Geometry check sheet. Reference: the model listing, model coordinates, mm. A direction names the side the tool comes from. Give positions to 0.01 mm unless a question says otherwise; leave off trailing zeros. Loops run counter-clockwise (first coordinate to the right, second up) from the corner with the lowest first, then second, coordinate; pieces in that order, holes last. Notation, with made-up numbers: (-18.5, 83.5) -> (37.5, 83.5) arc R12 cw to (37.5, 105.5) -> close; hole circle Ø1 at (8.25, 66). An arc over 180 degrees is marked (long way). Answer as a JSON object with one key per item and string values.
from build123d import *

# Parameters (mm, degrees)
BOSS_EXTRUDE1_DEPTH = 10
SKETCH4_R           = 1.45
CUT_EXTRUDE2_DEPTH  = 93.209340633
FILLET3_R           = 5
CHAMFER1_SIZE       = 3
FILLET1_R           = 5
FILLET2_R           = 5
CHAMFER2_SIZE       = 1.6
CUT_EXTRUDE1_DEPTH  = 165.519185811
CHAMFER3_SIZE       = 1.6


# Some blends are built 0.0001 mm under size
with BuildPart() as part:
    # Sketch2 → Boss-Extrude1 (new body)
    with BuildSketch(Plane.XY):
        Polygon((-44.75, 78), (-37.75, 78), (-37.75, -74), (37.75, -74), (37.75, 78), (44.75, 78), (44.75, -80), (-44.75, -80), align=None)
    extrude(amount=BOSS_EXTRUDE1_DEPTH)

    # Sketch4 → Cut-Extrude2 (cut, through all)
    with BuildSketch(Plane.XY.offset(10)):
        with Locations((-41.25, 68)):
            Circle(SKETCH4_R)
        with Locations(Location((41.25, 68, 0), (0, 0, 180))):
            Circle(SKETCH4_R)
    extrude(amount=-CUT_EXTRUDE2_DEPTH, mode=Mode.SUBTRACT)

    # Fillet3
    fillet3_edges = [part.edges().sort_by_distance(p)[0] for p in [
        (-37.75, -74, 5),
        (37.75, -74, 5),
    ]]
    fillet(fillet3_edges, radius=FILLET3_R)

    # Chamfer1
    # the kernel refuses this chamfer: 3 mm, written as the material it takes off along each edge
    with BuildSketch(Plane(origin=(37.75, -69, 10), x_dir=(0.9996219169112968, 0, 0.02749587661058619), z_dir=(0, 1, 0))) as chamfer1_piece_1:
        Polygon((CHAMFER1_SIZE * 0.999621916911, CHAMFER1_SIZE * 0.0274958766106), (-CHAMFER1_SIZE * 0.0274958766106, CHAMFER1_SIZE * 0.999621916911), (0, 0), align=None)
    extrude(amount=154.715048964, mode=Mode.SUBTRACT)
    with BuildSketch(Plane(origin=(-32.75, -74, 10), x_dir=(0, -0.9996219169112968, 0.02749587661058619), z_dir=(1, 0, 0))) as chamfer1_piece_2:
        Polygon((CHAMFER1_SIZE * 0.999621916911, CHAMFER1_SIZE * 0.0274958766106), (-CHAMFER1_SIZE * 0.0274958766106, CHAMFER1_SIZE * 0.999621916911), (0, 0), align=None)
    extrude(amount=65.5, mode=Mode.SUBTRACT)
    with BuildSketch(Plane(origin=(-37.75, 85.715048964, 10), x_dir=(0.027495876610586775, 0, -0.9996219169112968), z_dir=(0, -1, 0))) as chamfer1_piece_3:
        Polygon((CHAMFER1_SIZE * 0.999621916911, -CHAMFER1_SIZE * 0.0274958766106), (-CHAMFER1_SIZE * 0.0274958766106, -CHAMFER1_SIZE * 0.999621916911), (0, 0), align=None)
    extrude(amount=154.715048964, mode=Mode.SUBTRACT)
    with BuildSketch(Plane(origin=(32.75, -69, 10), x_dir=(0, -1, 0), z_dir=(-1, 0, 0))) as chamfer1_piece_4:
        Polygon((5 + CHAMFER1_SIZE, 0), (5, -CHAMFER1_SIZE), (5, 0), align=None)
    revolve(axis=Axis((32.75, -69, 10), (0, 0, 1)), revolution_arc=90, mode=Mode.SUBTRACT)
    with BuildSketch(Plane(origin=(-32.75, -69, 10), x_dir=(-1, 0, 0), z_dir=(0, 1, 0))) as chamfer1_piece_5:
        Polygon((5, -CHAMFER1_SIZE), (5 + CHAMFER1_SIZE, 0), (5, 0), align=None)
    revolve(axis=Axis((-32.75, -69, 10), (0, 0, 1)), revolution_arc=90, mode=Mode.SUBTRACT)

    # Fillet1
    fillet1_edges = [part.edges().sort_by_distance(p)[0] for p in [
        (44.75, 78, 5),
        (-44.75, 78, 5),
    ]]
    fillet(fillet1_edges, radius=FILLET1_R)

    # Fillet2
    fillet2_edges = [part.edges().sort_by_distance(p)[0] for p in [
        (44.75, -80, 5),
        (-44.75, -80, 5),
    ]]
    fillet(fillet2_edges, radius=FILLET2_R)

    # Chamfer2
    chamfer2_edges = [part.edges().sort_by_distance(p)[0] for p in [
        (38.75, 78, 0),
        (-44.75, -1, 0),
        (-43.285533906, 76.535533906, 0),
        (43.285533906, 76.535533906, 0),
        (-38.75, 78, 0),
        (44.75, -1, 0),
        (0, -80, 0),
        (-43.285533906, -78.535533906, 0),
        (43.285533906, -78.535533906, 0),
    ]]
    chamfer(chamfer2_edges, length=CHAMFER2_SIZE)

    # Sketch3 → Cut-Extrude1 (cut, through all)
    with BuildSketch(Plane.XZ.offset(80)):
        with BuildLine():
            Line((-14.35, 18.4), (14.35, 18.4))
            ThreePointArc((14.35, 18.4), (22.75, 10), (14.35, 1.6))
            Line((14.35, 1.6), (-14.35, 1.6))
            ThreePointArc((-14.35, 1.6), (-22.75, 10), (-14.35, 18.4))
        make_face()
    extrude(amount=-CUT_EXTRUDE1_DEPTH, mode=Mode.SUBTRACT)

    # Chamfer3
    chamfer3_edges = [part.edges().sort_by_distance(p)[0] for p in [
        (-19.11235236, -74, 3.080462443),
        (19.11235236, -74, 3.080462443),
        (0, -74, 1.6),
    ]]
    chamfer(chamfer3_edges, length=CHAMFER3_SIZE - 0.0001)  # a hair under: the kernel refuses the full size


solid = part.part
1) Depth check by flat-ended pin: P1, Ø2, axis at x = 5, z = 3, coming from the +Y side; P2, Ø4, axis at x = -41.25, y = 68, coming from the -Z side; P3, Ø5, axis at x = -6, y = -77.5, coming from the +Z side; P4, Ø6, axis at x = -28.5, z = 4, coming from the +Y side. Enter the tip coordinate at first touch or a pass-through.
Geometry check:
{"P1": "passes through", "P2": "stops at z = 0", "P3": "stops at z = 1.6", "P4": "stops at y = -74"}
2) Section check A-A on y = -30. Record the cut outline in (x, z), plus the area to 3 significant figures.
Geometry check:
{"outline": "(-44.75, 1.6) -> (-43.15, 0) -> (-37.75, 0) -> (-37.75, 7) -> (-40.75, 10) -> (-44.75, 10) -> close; (37.75, 0) -> (43.15, 0) -> (44.75, 1.6) -> (44.75, 10) -> (40.75, 10) -> (37.75, 7) -> close", "area": "128 mm2"}
3) Material ranges on line 1 along X through (y, z) = (68, 4.75); line 2 along X through (y, z) = (-12.5, 3.5); line 3 along X through (y, z) = (68, 7.5), recorded low to high. Write a range as from..to.
Geometry check:
{"line 1": "x = -44.75..-42.7, -39.8..-37.75, 37.75..39.8, 42.7..44.75", "line 2": "x = -44.75..-37.75, 37.75..44.75", "line 3": "x = -44.75..-42.7, -39.8..-38.25, 38.25..39.8, 42.7..44.75"}
4) Draft check along X on faces 6 (the face through (-43, -7, 10)), 7 (the face through (-44.75, -2, 6)), 8 (the face through (-28, -76, 9)), 9 (the face through (43.25, -78.57, 5.86)). Enter one of: pulls with the +X half, pulls with the -X half, needs draft (parallel to the pull), parting line crosses it, or undercut.
Geometry check:
{"face 6": "needs draft", "face 7": "pulls with the -X half", "face 8": "undercut", "face 9": "pulls with the +X half"}
5) Tool access check on faces 1 (the face through (-20, -74, 1)), 2 (the face through (0, -78, 1.6)), 3 (the face through (-20.132, -75.144, 3.293)), 4 (the face through (42.63, -77.82, 0.63)), 5 (the face through (42.7, 67.94, 5.07)). Record the directions out of +Z, -Z, +X, -X, +Y, -Y that give a thin tool (end or side, any length) a straight path to the whole face; none if there is none.
Geometry check:
{"face 1": "+Z, -Z, +Y", "face 2": "+Z, +Y, -Y", "face 3": "+Z, +Y", "face 4": "-Z, +X, -Y", "face 5": "+Z, -Z"}
